Geometry check sheet. Reference: drawing and pictorial views, mm from the part's lowest x, y, z. A direction names the side the tool comes from. Coordinates: 2 decimals unless noted, no trailing zeros. Write each loop counter-clockwise with the first axis right and the second up, starting at its lowest first coordinate (ties: lowest second). Pieces come first, ordered by that corner, then holes. Notation, with made-up numbers: (71, 80.5) - (120, 80.5) arc R26 ccw to (120, 96.5) - close; hole circle Ø1 at (86.25, 16.25). An arc over 180 degrees is marked (long way). Answer as a JSON object with one key per item and string values. Group by question number.
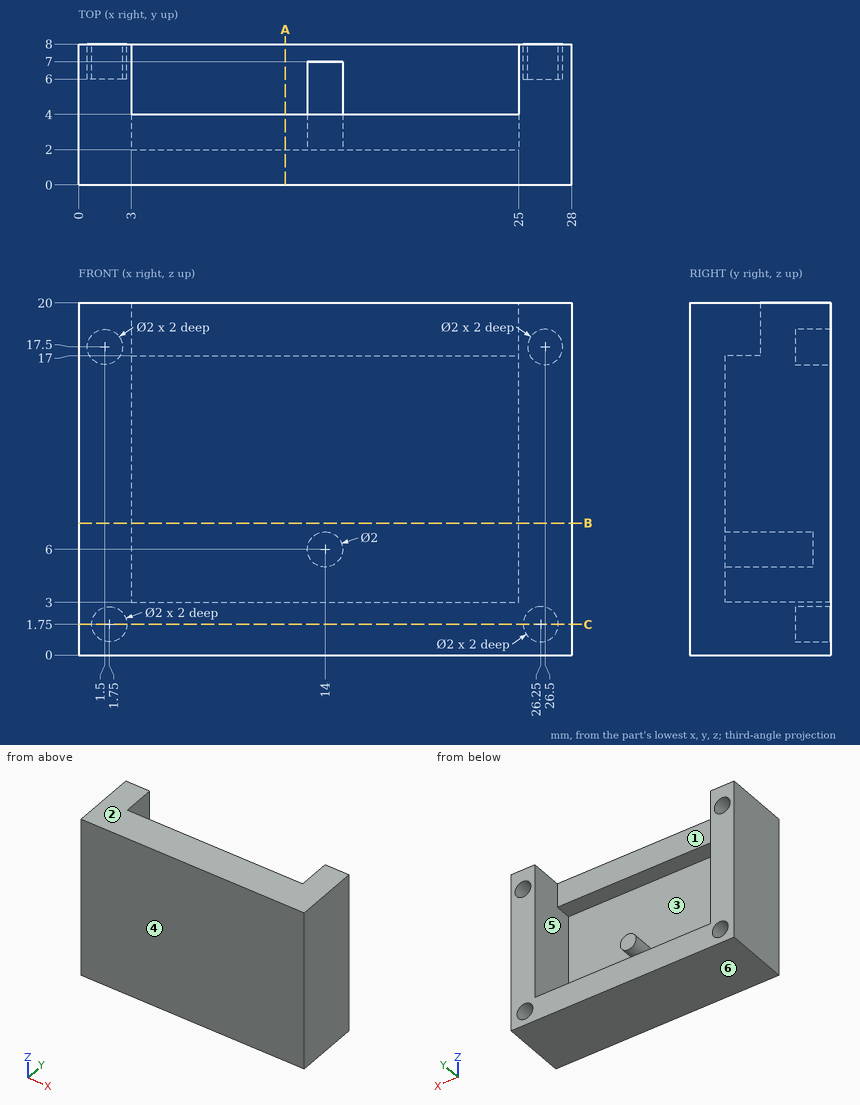
(1) Section check B-B (z = 7.5). Record the cut outline in (x, y).
(2) Gauge pin test, flat ends, axial feed: pin 1 (2.5 mm diameter, centred on x = 9.5, z = 19, fed in from +Y); pin 2 (4 mm diameter, centred on x = 19.5, z = 6, fed in from -Y); pin 3 (2 mm diameter, centred on x = 14, z = 6, fed in from +Y); pin 4 (3 mm diameter, centred on x = 22.5, z = 8.5, fed in from +Y). Record the tip position at first contact, or that the pin passes through.
(3) Section check C-C (z = 1.75). Record the cut outline in (x, y).
(4) Section check A-A (x = 11.75). Record the cut outline in (y, z).
(5) Material ranges on L1, parallel to X at y = 7.25, z = 1.75; L2, parallel to X at y = 6.7, z = 17.5; L3, parallel to X at y = 6.5, z = 11.5, recorded low to high. Write a range as [from, to].
(6) Draft check along Z on the marked faces 3, 4, 5 and 6. Enter one of: +Z half, -Z half, draft (parallel to the pull), parting line (faces both ways), or undercut.
(7) Set-up check for the marked faces 1 and 2: record each of +Z, -Z, +X, -X, +Y, -Y from which the full face is reachable in a straight line by a thin tool's end or side.
Conclusion:
{
 "1": {"outline": "(0, 0) - (28, 0) - (28, 8) - (25, 8) - (25, 2) - (3, 2) - (3, 8) - (0, 8) - close"},
 "2": {"pin 1": "stops at y = 4", "pin 2": "stops at y = 0", "pin 3": "stops at y = 7", "pin 4": "stops at y = 2"},
 "3": {"outline": "(0, 0) - (28, 0) - (28, 8) - (27.25, 8) - (27.25, 6) - (25.25, 6) - (25.25, 8) - (2.75, 8) - (2.75, 6) - (0.75, 6) - (0.75, 8) - (0, 8) - close"},
 "4": {"outline": "(0, 0) - (8, 0) - (8, 3) - (2, 3) - (2, 17) - (4, 17) - (4, 20) - (0, 20) - close"},
 "5": {"L1": "x = [0, 0.75], [2.75, 25.25], [27.25, 28]", "L2": "x = [0, 0.5], [2.5, 3], [25, 25.5], [27.5, 28]", "L3": "x = [0, 3], [25, 28]"},
 "6": {"face 3": "undercut", "face 4": "draft", "face 5": "undercut", "face 6": "-Z half"},
 "7": {"face 1": "+Z, +Y", "face 2": "+Z, +X, -X, +Y, -Y"}
}
